```python
from build123d import *

# Parameters (mm, degrees)
F0_W     = 150
F0_H     = 85
F0_R     = 3.4
F0_R_2   = 1.45
F0_R_3   = 3.44
F0_R_4   = 6
F0_W_2   = 71
F0_H_2   = 24
F0_R_5   = 4.675
F1_DEPTH = 2


with BuildPart() as f1:
    # F0 (on Front) → F1 (new body)
    with BuildSketch(Plane.XZ):
        with Locations((-152.851582, -79.104053)):
            Rectangle(F0_W, F0_H)
        with Locations((-206.544898, -101.604053)):
            Circle(F0_R, mode=Mode.SUBTRACT)
        with Locations((-208.544898, -83.604053)):
            Circle(F0_R_2, mode=Mode.SUBTRACT)
        with Locations((-135.544898, -101.604053)):
            Circle(F0_R_3, mode=Mode.SUBTRACT)
        with Locations((-106.69824, -101.604053)):
            Circle(F0_R_4, mode=Mode.SUBTRACT)
        with Locations((-133.544898, -83.604053)):
            Circle(F0_R_2, mode=Mode.SUBTRACT)
        with Locations((-171.044898, -68.604053)):
            Rectangle(F0_W_2, F0_H_2, mode=Mode.SUBTRACT)
        with Locations((-208.544898, -52.604053)):
            Circle(F0_R_2, mode=Mode.SUBTRACT)
        with Locations((-106.69824, -68.604053)):
            Circle(F0_R_5, mode=Mode.SUBTRACT)
        with Locations((-133.544898, -52.604053)):
            Circle(F0_R_2, mode=Mode.SUBTRACT)
    extrude(amount=F1_DEPTH)


solid = f1.part
```
Verification items for the finished model (mm, model axes). Coordinates: 2 decimals unless noted, no trailing zeros. Loops run counter-clockwise (first coordinate to the right, second up) from the corner with the lowest first, then second, coordinate; pieces in that order, holes last. Notation, with made-up numbers: (87.25, 43) -> (112.25, 43) arc R18 cw to (112.25, 49) -> close; hole circle Ø10 at (51, -35.5). An arc over 180 degrees is marked (long way). Answer in a Markdown table with one row per item. Add a question column.
1. Section check A-A, the plane z = -79. Enter the section's corners in (x, y).
2. Section check D-D, the plane y = -1.45. Give the number of separate pieces and of enclosed holes in the cut face, then the cut area to 3 significant figures.
3. Section check B-B, the plane x = -184.5. Enter the section's corners in (y, z).
4. Section check C-C, the plane x = -107. Enter the section's corners in (y, z).
5. Material ranges on probe 1 along X at (y, z) = (-1.5, -57.5); probe 2 along X at (y, z) = (-1.9, -84.5); probe 3 along X at (y, z) = (-0.2, -65), recorded low to high. Write a range as [from, to].
6. Depth check by flat-ended pin: P1, Ø3.5, axis at x = -133.54, z = -83.6, coming from the +Y side; P2, Ø4, axis at x = -135.54, z = -101.6, coming from the +Y side. Enter the tip coordinate at first touch or a pass-through.
7. Draft check along Z on faces 1 (the face through (-107.31, -0.99, -63.97)), 2 (the face through (-154, -2, -88)). Enter one of: +Z half, -Z half, draft (parallel to the pull), parting line (faces both ways), or undercut.
Derived:
| question | item | result |
|---|---|---|
| 1 | outline | (-227.85, -2) -> (-206.54, -2) -> (-206.54, 0) -> (-227.85, 0) -> close; (-135.54, -2) -> (-77.85, -2) -> (-77.85, 0) -> (-135.54, 0) -> close |
| 2 | separate pieces | 1 |
| 2 | enclosed holes | 9 |
| 2 | area | 10,800 mm² |
| 3 | outline | (-2, -121.6) -> (0, -121.6) -> (0, -80.6) -> (-2, -80.6) -> close; (-2, -56.6) -> (0, -56.6) -> (0, -36.6) -> (-2, -36.6) -> close |
| 4 | outline | (-2, -121.6) -> (0, -121.6) -> (0, -107.6) -> (-2, -107.6) -> close; (-2, -95.61) -> (0, -95.61) -> (0, -73.27) -> (-2, -73.27) -> close; (-2, -63.94) -> (0, -63.94) -> (0, -36.6) -> (-2, -36.6) -> close |
| 5 | probe 1 | x = [-227.85, -206.54], [-135.54, -77.85] |
| 5 | probe 2 | x = [-227.85, -209.68], [-207.4, -134.68], [-132.4, -77.85] |
| 5 | probe 3 | x = [-227.85, -206.54], [-135.54, -109.68], [-103.72, -77.85] |
| 6 | P1 | stops at y = 0 |
| 6 | P2 | passes through |
| 7 | face 1 | undercut |
| 7 | face 2 | draft |
